from build123d import *
from build123d.topology import SkipClean

# Parameters (mm, degrees)
BOSS_EXTRUDE1_DEPTH = 15
BOSS_EXTRUDE2_START = -220
BOSS_EXTRUDE2_DEPTH = 10


with BuildPart() as part:
    # Sketch1 → Revolve2 (revolve)
    with BuildSketch(Plane.XY, mode=Mode.PRIVATE) as revolve2_sk:
        Polygon((-185, 0), (-185, 12), (-135, 12), (-135, 20), (-70, 20), (-70, 35), (-80, 35), (-80, 50), (140, 50), (140, 35), (130, 35), (130, 20), (160, 20), (160, 12), (185, 12), (185, 0), align=None)
    revolve(revolve2_sk.sketch.rotate(Axis((-185, 0, 0), (1, 0, 0)), 180), axis=Axis((-185, 0, 0), (1, 0, 0)))

    # Sketch4 → Boss-Extrude1 (add)
    with SkipClean():  # the faces are left unmerged after this step: merging them gives an invalid solid
        with BuildSketch(Plane.ZY.offset(80)):
            with BuildLine():
                Line((-1.25, 49.984372558), (-1.25, 34.977671449))
                ThreePointArc((-1.25, 34.977671449), (0, 35), (1.25, 34.977671449))
                Line((1.25, 34.977671449), (1.25, 49.984372558))
                ThreePointArc((1.25, 49.984372558), (0, 50), (-1.25, 49.984372558))
            make_face()
            with BuildLine():
                Line((34.460405313, 36.228172265), (23.849065195, 25.616832148))
                ThreePointArc((23.849065195, 25.616832148), (24.748737342, 24.748737342), (25.616832148, 23.849065195))
                Line((25.616832148, 23.849065195), (36.228172265, 34.460405313))
                ThreePointArc((36.228172265, 34.460405313), (35.355339059, 35.355339059), (34.460405313, 36.228172265))
            make_face()
            with BuildLine():
                Line((49.984372558, 1.25), (34.977671449, 1.25))
                ThreePointArc((34.977671449, 1.25), (35, 0), (34.977671449, -1.25))
                Line((34.977671449, -1.25), (49.984372558, -1.25))
                ThreePointArc((49.984372558, -1.25), (50, 0), (49.984372558, 1.25))
            make_face()
            with BuildLine():
                Line((36.228172265, -34.460405313), (25.616832148, -23.849065195))
                ThreePointArc((25.616832148, -23.849065195), (24.748737342, -24.748737342), (23.849065195, -25.616832148))
                Line((23.849065195, -25.616832148), (34.460405313, -36.228172265))
                ThreePointArc((34.460405313, -36.228172265), (35.355339059, -35.355339059), (36.228172265, -34.460405313))
            make_face()
            with BuildLine():
                Line((1.25, -49.984372558), (1.25, -34.977671449))
                ThreePointArc((1.25, -34.977671449), (0, -35), (-1.25, -34.977671449))
                Line((-1.25, -34.977671449), (-1.25, -49.984372558))
                ThreePointArc((-1.25, -49.984372558), (0, -50), (1.25, -49.984372558))
            make_face()
            with BuildLine():
                Line((-34.460405313, -36.228172265), (-23.849065195, -25.616832148))
                ThreePointArc((-23.849065195, -25.616832148), (-24.748737342, -24.748737342), (-25.616832148, -23.849065195))
                Line((-25.616832148, -23.849065195), (-36.228172265, -34.460405313))
                ThreePointArc((-36.228172265, -34.460405313), (-35.355339059, -35.355339059), (-34.460405313, -36.228172265))
            make_face()
            with BuildLine():
                Line((-49.984372558, -1.25), (-34.977671449, -1.25))
                ThreePointArc((-34.977671449, -1.25), (-35, 0), (-34.977671449, 1.25))
                Line((-34.977671449, 1.25), (-49.984372558, 1.25))
                ThreePointArc((-49.984372558, 1.25), (-50, 0), (-49.984372558, -1.25))
            make_face()
            with BuildLine():
                Line((-36.228172265, 34.460405313), (-25.616832148, 23.849065195))
                ThreePointArc((-25.616832148, 23.849065195), (-24.748737342, 24.748737342), (-23.849065195, 25.616832148))
                Line((-23.849065195, 25.616832148), (-34.460405313, 36.228172265))
                ThreePointArc((-34.460405313, 36.228172265), (-35.355339059, 35.355339059), (-36.228172265, 34.460405313))
            make_face()
        extrude(amount=BOSS_EXTRUDE1_DEPTH)

    # Sketch4_2 → Boss-Extrude2 (add)
    with SkipClean():  # the faces are left unmerged after this step: merging them gives an invalid solid
        with BuildSketch(Plane.ZY.offset(80).offset(BOSS_EXTRUDE2_START)):
            with BuildLine():
                ThreePointArc((1.25, 49.984372558), (0, 50), (-1.25, 49.984372558))
                Line((-1.25, 49.984372558), (-1.25, 34.977671449))
                ThreePointArc((-1.25, 34.977671449), (0, 35), (1.25, 34.977671449))
                Line((1.25, 34.977671449), (1.25, 49.984372558))
            make_face()
            with BuildLine():
                Line((-23.849065195, 25.616832148), (-34.460405313, 36.228172265))
                ThreePointArc((-34.460405313, 36.228172265), (-35.355339059, 35.355339059), (-36.228172265, 34.460405313))
                Line((-36.228172265, 34.460405313), (-25.616832148, 23.849065195))
                ThreePointArc((-25.616832148, 23.849065195), (-24.748737342, 24.748737342), (-23.849065195, 25.616832148))
            make_face()
            with BuildLine():
                ThreePointArc((36.228172265, 34.460405313), (35.355339059, 35.355339059), (34.460405313, 36.228172265))
                Line((34.460405313, 36.228172265), (23.849065195, 25.616832148))
                ThreePointArc((23.849065195, 25.616832148), (24.748737342, 24.748737342), (25.616832148, 23.849065195))
                Line((25.616832148, 23.849065195), (36.228172265, 34.460405313))
            make_face()
            with BuildLine():
                Line((-34.977671449, 1.25), (-49.984372558, 1.25))
                ThreePointArc((-49.984372558, 1.25), (-50, 0), (-49.984372558, -1.25))
                Line((-49.984372558, -1.25), (-34.977671449, -1.25))
                ThreePointArc((-34.977671449, -1.25), (-35, 0), (-34.977671449, 1.25))
            make_face()
            with BuildLine():
                ThreePointArc((49.984372558, -1.25), (50, 0), (49.984372558, 1.25))
                Line((49.984372558, 1.25), (34.977671449, 1.25))
                ThreePointArc((34.977671449, 1.25), (35, 0), (34.977671449, -1.25))
                Line((34.977671449, -1.25), (49.984372558, -1.25))
            make_face()
            with BuildLine():
                Line((-25.616832148, -23.849065195), (-36.228172265, -34.460405313))
                ThreePointArc((-36.228172265, -34.460405313), (-35.355339059, -35.355339059), (-34.460405313, -36.228172265))
                Line((-34.460405313, -36.228172265), (-23.849065195, -25.616832148))
                ThreePointArc((-23.849065195, -25.616832148), (-24.748737342, -24.748737342), (-25.616832148, -23.849065195))
            make_face()
            with BuildLine():
                ThreePointArc((34.460405313, -36.228172265), (35.355339059, -35.355339059), (36.228172265, -34.460405313))
                Line((36.228172265, -34.460405313), (25.616832148, -23.849065195))
                ThreePointArc((25.616832148, -23.849065195), (24.748737342, -24.748737342), (23.849065195, -25.616832148))
                Line((23.849065195, -25.616832148), (34.460405313, -36.228172265))
            make_face()
            with BuildLine():
                Line((-1.25, -34.977671449), (-1.25, -49.984372558))
                ThreePointArc((-1.25, -49.984372558), (0, -50), (1.25, -49.984372558))
                Line((1.25, -49.984372558), (1.25, -34.977671449))
                ThreePointArc((1.25, -34.977671449), (0, -35), (-1.25, -34.977671449))
            make_face()
        extrude(amount=-BOSS_EXTRUDE2_DEPTH)


solid = part.part
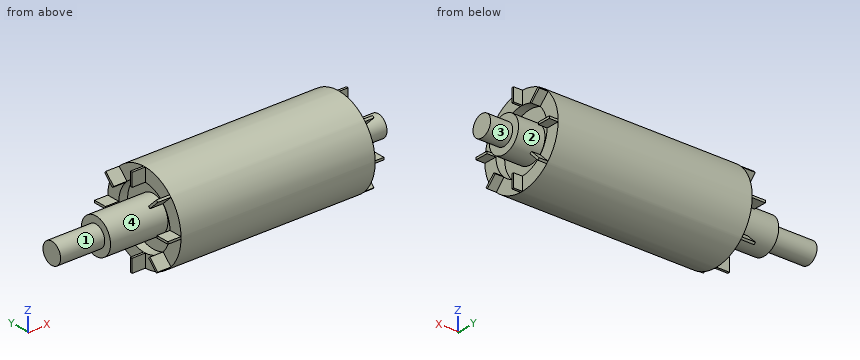
Here's how the part is built. I have some questions about the finished solid (model axes, mm). Face numbers are marked on the shaded views. A direction names the side the tool comes from. Round coordinates to 2 decimals unless told otherwise and drop trailing zeros. Order: outer loops, then holes, each group sorted by start corner. A loop starts at its lowest first (then second) coordinate and runs counter-clockwise, first axis right, second up. Notation, with made-up numbers: M -29.75,-10.75 L -25.75,-10.75 A21 ccw -25.75,5.25 Z; hole C 61.5,6.5 d5. An arc over 180 degrees is marked long. One line per question, with ' | ' between items.
1) On a 3-axis mill with a long thin cutter (end or side, diameter ignored), from which of +Z, -Z, +X, -X, +Y, -Y can I reach the whole of each face in a straight line? I mean the marked faces 3 and 4. Say none if no direction works.
Checked values:
face 3: +X | face 4: -X
2) Imagine slicing it at B-B, the plane y = -15.5. Write out the boundary of the cut face in (x, z), plus the area to 3 significant figures.
Checked values:
outline: M -135,-12.64 L -70,-12.64 L -70,-31.38 L -80,-31.38 L -80,-47.54 L 140,-47.54 L 140,-31.38 L 130,-31.38 L 130,-12.64 L 160,-12.64 L 160,12.64 L 130,12.64 L 130,31.38 L 140,31.38 L 140,47.54 L -80,47.54 L -80,31.38 L -70,31.38 L -70,12.64 L -135,12.64 Z | area: 22,100 mm²
3) I need wall thicknesses on line 1 (Z direction, x = -75.5, y = 0); line 2 (X direction, y = 11, z = -25); line 3 (Y direction, x = -49.5, z = 1.5). Which ranges of each line are inside material? Lowest first, please.
Checked values:
line 1: z = -50 to -35, -20 to 20, 35 to 50 | line 2: x = -70 to 130 | line 3: y = -49.98 to 49.98
4) We'd pull the mould along Z, two halves only. Please class the marked faces 1 and 2: released by +Z, released by -Z, zero draft, split by the parting line, or undercut.
Checked values:
face 1: split by the parting line | face 2: undercut
5) Imagine slicing it at A-A, the plane z = 29. Write out the boundary of the cut face in (x, y).
Checked values:
outline: M -95,-30.77 L -80,-30.77 L -80,-40.73 L 140,-40.73 L 140,-30.77 L 150,-30.77 L 150,-27.23 L 140,-27.23 L 140,-19.6 L 130,-19.6 L 130,19.6 L 140,19.6 L 140,27.23 L 150,27.23 L 150,30.77 L 140,30.77 L 140,40.73 L -80,40.73 L -80,30.77 L -95,30.77 L -95,27.23 L -80,27.23 L -80,19.6 L -70,19.6 L -70,-19.6 L -80,-19.6 L -80,-27.23 L -95,-27.23 Z
6) I'm going to push flat-ended pins straight in: pin 1 Ø1 at (y, z) = (-15, 15.5) entering from -X; pin 2 Ø4 at (y, z) = (31.5, -40) entering from +X; pin 3 Ø1.5 at (x, y) = (-54.5, -21.5) entering from +Z. Where does each tip first touch, or does it pass through?
Checked values:
pin 1: stops at x = -70 | pin 2: stops at x = 140 | pin 3: stops at z = 45.49
